```python
from build123d import *

# Parameters (mm, degrees)
SKETCH1_W           = 270
SKETCH1_H           = 80
BOSS_EXTRUDE1_DEPTH = 6
SKETCH2_R           = 3.1
CUT_EXTRUDE1_DEPTH  = 141.929060169
FILLET1_R           = 10
CUT_EXTRUDE2_DEPTH  = 10
FILLET2_R           = 10


with BuildPart() as part:
    # Sketch1 → Boss-Extrude1 (new body)
    with BuildSketch(Plane.XY):
        Rectangle(SKETCH1_W, SKETCH1_H)
    extrude(amount=BOSS_EXTRUDE1_DEPTH)

    # Sketch2 → Cut-Extrude1 (cut, through all)
    with BuildSketch(Plane.XY.offset(6)):
        with Locations((-79, 25)):
            Circle(SKETCH2_R)
        with Locations((119, 25)):
            Circle(SKETCH2_R)
        with Locations((119, -25)):
            Circle(SKETCH2_R)
        with Locations((-92.21, -25)):
            Circle(SKETCH2_R)
    extrude(amount=-CUT_EXTRUDE1_DEPTH, mode=Mode.SUBTRACT)

    # Fillet1
    fillet1_edges = [part.edges().sort_by_distance(p)[0] for p in [
        (135, -40, 3),
        (-135, -40, 3),
        (-135, 40, 3),
        (135, 40, 3),
    ]]
    fillet(fillet1_edges, radius=FILLET1_R)

    # Sketch3 → Cut-Extrude2 (cut)
    with BuildSketch(Plane.XY.offset(6)):
        Polygon((-112.21, -40), (-154.206287839, 3.47324229), (-156.168985045, -56.555388838), (-112.21, -57.992672605), align=None)
    extrude(amount=-CUT_EXTRUDE2_DEPTH, mode=Mode.SUBTRACT)

    # Fillet2
    fillet2_edges = [part.edges().sort_by_distance(p)[0] for p in [
        (-135, -16.408505543, 3),
        (-112.21, -40, 3),
    ]]
    fillet(fillet2_edges, radius=FILLET2_R)


solid = part.part
```
The listing builds one solid part. Answer for the finished solid, in the listing's coordinates (mm). Give positions to 0.01 mm unless a question says otherwise; leave off trailing zeros. Loops run counter-clockwise (first coordinate to the right, second up) from the corner with the lowest first, then second, coordinate; pieces in that order, holes last. Notation, with made-up numbers: (-20.5, 79) - (29.5, 79) arc R10 cw to (29.5, 95) - close; hole circle Ø2 at (33, 17). An arc over 180 degrees is marked (long way). Return JSON: item names as keys, results as strings. Group by question number.
1. Determine the mould class of faces 1 (the flat face through (135, 0, 3)), 2 (the cylindrical face through (121.957, 25.931, 3.042)), 3 (the cylindrical face through (121.957, -24.069, 3.042)), 4 (the flat face through (7, -40, 3)) for opening direction X: pulls with the +X half, pulls with the -X half, needs draft (parallel to the pull), parting line crosses it, or undercut.
2. Find section D-D (x = -92.21). Write down the section's boundary in (y, z).
3. Find section A-A (x = 119). Write down the section's boundary in (y, z), then the cut area to 3 significant figures.
4. Straight lines are drawn through the part: line 1 (Y direction, x = 119, z = 2.45); line 2 (Y direction, x = -92.21, z = 3.05); line 3 (X direction, y = -13.5, z = 3.1). For each, find the intervals that lie inside material, in ascending order. Write a range as [from, to].
5. Find section C-C (y = 25). Write down the section's boundary in (x, z), then the cut area to 3 significant figures.
6. Find section B-B (z = 1.85). Write down the section's boundary in (x, y).
Verdict:
{
 "1": {"face 1": "pulls with the +X half", "face 2": "undercut", "face 3": "undercut", "face 4": "needs draft"},
 "2": {"outline": "(-40, 0) - (-28.1, 0) - (-28.1, 6) - (-40, 6) - close; (-21.9, 0) - (40, 0) - (40, 6) - (-21.9, 6) - close"},
 "3": {"outline": "(-40, 0) - (-28.1, 0) - (-28.1, 6) - (-40, 6) - close; (-21.9, 0) - (21.9, 0) - (21.9, 6) - (-21.9, 6) - close; (28.1, 0) - (40, 0) - (40, 6) - (28.1, 6) - close", "area": "406 mm^2"},
 "4": {"line 1": "y = [-40, -28.1], [-21.9, 21.9], [28.1, 40]", "line 2": "y = [-40, -28.1], [-21.9, 40]", "line 3": "x = [-134.94, 135]"},
 "5": {"outline": "(-135, 0) - (-82.1, 0) - (-82.1, 6) - (-135, 6) - close; (-75.9, 0) - (115.9, 0) - (115.9, 6) - (-75.9, 6) - close; (122.1, 0) - (135, 0) - (135, 6) - (122.1, 6) - close", "area": "1,550 mm^2"},
 "6": {"outline": "(-135, -12.37) arc R10 ccw to (-132.19, -19.32) - (-115.16, -36.95) arc R10 ccw to (-107.97, -40) - (125, -40) arc R10 ccw to (135, -30) - (135, 30) arc R10 ccw to (125, 40) - (-125, 40) arc R10 ccw to (-135, 30) - close; hole circle Ø6.2 at (-92.21, -25); hole circle Ø6.2 at (-79, 25); hole circle Ø6.2 at (119, -25); hole circle Ø6.2 at (119, 25)"}
}
